Check sheet for the modelled part. Datum: model origin and axes. Units: mm. Face numbers are marked on the shaded views. A direction names the side the tool comes from. Round coordinates to 2 decimals unless told otherwise and drop trailing zeros. Write each loop counter-clockwise with the first axis right and the second up, starting at its lowest first coordinate (ties: lowest second). Pieces come first, ordered by that corner, then holes. Notation, with made-up numbers: (84.25, 59) - (123.25, 59) arc R10 cw to (123.25, 65) - close; hole circle Ø4 at (72.25, -37.5). An arc over 180 degrees is marked (long way). Use one line per item in the form item = value. Start each with the question number.
1) Set-up check for the marked faces 4, 5, 6 and 7: record each of +Z, -Z, +X, -X, +Y, -Y from which the full face is reachable in a straight line by a thin tool's end or side.
2) Draft check along Z on the marked faces 1, 2 and 3. Enter one of: +Z half, -Z half, draft (parallel to the pull), parting line (faces both ways), or undercut.
3) Scan lines: probe 1 along Y at (x, z) = (9, -7.5); probe 2 along Z at (x, y) = (8.25, -28.5); probe 3 along Y at (x, z) = (9.5, -18). Record each from-to range of solid material in increasing order.
4) Gauge pin test, flat ends, axial feed: P1, Ø4.5, axis at x = 10.5, y = -19.5, coming from the +Z side; P2, Ø1.6, axis at y = -25, z = -37.5, coming from the +X side; P3, Ø5, axis at x = 11.5, z = -32, coming from the +Y side; P4, Ø2, axis at x = 5, y = -27, coming from the -Z side. Record the tip position at first contact, or that the pin passes through.
5) Section check C-C (y = 6.5). Record the boundary of the cut face in (x, z).
6) Section check A-A (y = -25). Count the separate pieces of the cut face and the enclosed holes in it, then the cut area to 3 significant figures.
7) Section check B-B (z = -7.5). Record the boundary of the cut face in (x, y), then the cut area to 3 significant figures.
from build123d import *

# Parameters (mm, degrees)
SKETCH_3_W               = 45
SKETCH_3_H               = 5
EXTRUDE_2_DEPTH          = 15
SKETCH_4_W               = 15
SKETCH_4_H               = 5
EXTRUDE_3_DEPTH          = 10
SKETCH_6_R               = 1.25
CUT_EXTRUDE_3_DEPTH      = 50
FILLET_3_R               = 3
SKETCH_7_W               = 15
SKETCH_7_H               = 5
EXTRUDE_4_DEPTH          = 40
FILLET_4_R               = 10
FILLET_5_R               = 5
FILLET_6_R               = 1
FILLET_7_SIZE            = 10
FILLET_7_SIZE_2          = 2.5
SKETCH_8_R               = 1
CUT_EXTRUDE_4_DEPTH      = 40
MIRROR_2_COPY_1_SKETCH_R = 1
MIRROR_2_COPY_1_DEPTH    = 40
MIRROR_2_COPY_2_SKETCH_R = 1
MIRROR_2_COPY_2_DEPTH    = 40
MIRROR_2_COPY_3_SKETCH_R = 1
MIRROR_2_COPY_3_DEPTH    = 40


with BuildPart() as part:
    # 草图3 → 凸台-拉伸2 (new body)
    with BuildSketch(Plane(origin=(0, 0, 0), x_dir=(0, 0, -1), z_dir=(1, 0, 0))):
        with Locations((22.5, 2.5)):
            Rectangle(SKETCH_3_W, SKETCH_3_H)
    extrude(amount=EXTRUDE_2_DEPTH)

    # 草图4 → 凸台-拉伸3 (add)
    with BuildSketch(Plane(origin=(0, 5, 0), x_dir=(1, 0, 0), z_dir=(0, 1, 0))):
        with Locations((7.5, 42.5)):
            Rectangle(SKETCH_4_W, SKETCH_4_H)
        with Locations((7.5, 2.5)):
            Rectangle(SKETCH_4_W, SKETCH_4_H)
    extrude(amount=EXTRUDE_3_DEPTH)

    # 草图6 → 切除-拉伸3 (cut)
    with BuildSketch(Plane.XY):
        with Locations((3.5, 10)):
            Circle(SKETCH_6_R)
        with Locations((11.5, 10)):
            Circle(SKETCH_6_R)
    extrude(amount=-CUT_EXTRUDE_3_DEPTH, mode=Mode.SUBTRACT)

    # 圆角3
    fillet_3_edges = [part.edges().sort_by_distance(p)[0] for p in [
        (0, 15, -42.5),
        (15, 15, -42.5),
        (0, 15, -2.5),
        (15, 15, -2.5),
    ]]
    fillet(fillet_3_edges, radius=FILLET_3_R)

    # 草图7 → 凸台-拉伸4 (add)
    with BuildSketch(Plane(origin=(0, 0, 0), x_dir=(-1, 0, 0), z_dir=(0, -1, 0))):
        with Locations((-7.5, 27.5)):
            Rectangle(SKETCH_7_W, SKETCH_7_H)
        with Locations((-7.5, 17.5)):
            Rectangle(SKETCH_7_W, SKETCH_7_H)
        with Locations((-7.5, 37.5)):
            Rectangle(SKETCH_7_W, SKETCH_7_H)
        with Locations((-7.5, 7.5)):
            Rectangle(SKETCH_7_W, SKETCH_7_H)
    extrude(amount=EXTRUDE_4_DEPTH)

    # 圆角4
    # the kernel refuses this fillet: 10 mm, written as the material it adds along each edge
    with BuildSketch(Plane(origin=(0, 0, -5), x_dir=(0, 0, 1), z_dir=(1, 0, 0)), Plane(origin=(15, 0, -40), x_dir=(0, 0, -1), z_dir=(-1, 0, 0))) as fillet_4_piece_1:
        with BuildLine():
            CenterArc((10, 8.660254038), FILLET_4_R, 180, 60)
            Line((0, 8.660254038), (-0.2, 8.660254038))
            Line((-0.2, 8.660254038), (-0.2, 0))
            Line((-0.2, 0), (0, -0.2))
            ThreePointArc((0, -0.2), (2.5, -0.2), (4.9, -0.173205081))
            Line((4.9, -0.173205081), (5, 0))
        make_face()
    extrude(amount=15)

    # 圆角5
    fillet_5_edges = [part.edges().sort_by_distance(p)[0] for p in [
        (7.5, 0, -45),
        (7.5, 0, 0),
    ]]
    fillet(fillet_5_edges, radius=FILLET_5_R)

    # 圆角6
    fillet_6_edges = [part.edges().sort_by_distance(p)[0] for p in [
        (7.5, -40, -15),
        (7.5, -40, -20),
        (7.5, -40, -35),
        (7.5, -40, -40),
        (7.5, -40, -5),
        (7.5, -40, -10),
        (7.5, -40, -25),
        (7.5, -40, -30),
    ]]
    fillet(fillet_6_edges, radius=FILLET_6_R)

    # 圆角7
    # an asymmetric fillet: 10, 2.5 mm, written as the material it adds along each edge
    with BuildSketch(Plane(origin=(15, 0, -10), x_dir=(0, -1, 0), z_dir=(-1, 0, 0)), Plane(origin=(15, 0, -20), x_dir=(0, -1, 0), z_dir=(-1, 0, 0)), Plane(origin=(15, 0, -30), x_dir=(0, -1, 0), z_dir=(-1, 0, 0)), Plane(origin=(0, 0, -35), x_dir=(0, -1, 0), z_dir=(1, 0, 0))) as fillet_7_piece_1:
        with BuildLine():
            Bezier((FILLET_7_SIZE, 0), (0, 0), (0, -FILLET_7_SIZE_2), weights=[1, 0.707106781, 1])
            Line((0, -FILLET_7_SIZE_2), (0, 0))
            Line((0, 0), (FILLET_7_SIZE, 0))
        make_face()
    extrude(amount=15)
    with BuildSketch(Plane(origin=(0, 0, -15), x_dir=(0, 0, 1), z_dir=(1, 0, 0)), Plane(origin=(0, 0, -25), x_dir=(0, 0, 1), z_dir=(1, 0, 0))) as fillet_7_piece_2:
        with BuildLine():
            Bezier((FILLET_7_SIZE_2, 0), (0, 0), (0, FILLET_7_SIZE), weights=[1, 0.707106781, 1])
            Line((0, FILLET_7_SIZE), (0, 0))
            Line((0, 0), (FILLET_7_SIZE_2, 0))
        make_face()
    extrude(amount=15)

    # 草图8 → 切除-拉伸4 (cut)
    with BuildSketch(Plane.ZY):
        with Locations((-27.5, -15)):
            Circle(SKETCH_8_R)
        with Locations((-27.5, -20)):
            Circle(SKETCH_8_R)
        with Locations((-27.5, -25)):
            Circle(SKETCH_8_R)
        with Locations((-27.5, -30)):
            Circle(SKETCH_8_R)
        with Locations((-27.5, -35)):
            Circle(SKETCH_8_R)
    cut_extrude_4 = extrude(amount=-CUT_EXTRUDE_4_DEPTH, mode=Mode.SUBTRACT)

    # 镜向1: 切除-拉伸4 across plane
    add(cut_extrude_4.mirror(Plane(origin=(0, 0, -32.5), x_dir=(1, 0, 0), z_dir=(0, 0, -1))), mode=Mode.SUBTRACT)

    # 镜向1 at the second plane: 切除-拉伸4 across plane
    add(cut_extrude_4.mirror(Plane(origin=(0, 0, -22.5), x_dir=(1, 0, 0), z_dir=(0, 0, -1))), mode=Mode.SUBTRACT)

    # 镜向2 copy 1 sketch → 镜向2 copy 1 (cut)
    with BuildSketch(Plane(origin=(0, 0, 20), x_dir=(0, 0, 1), z_dir=(-1, 0, 0))):
        with Locations((-27.5, -15)):
            Circle(MIRROR_2_COPY_1_SKETCH_R)
        with Locations((-27.5, -20)):
            Circle(MIRROR_2_COPY_1_SKETCH_R)
        with Locations((-27.5, -25)):
            Circle(MIRROR_2_COPY_1_SKETCH_R)
        with Locations((-27.5, -30)):
            Circle(MIRROR_2_COPY_1_SKETCH_R)
        with Locations((-27.5, -35)):
            Circle(MIRROR_2_COPY_1_SKETCH_R)
    extrude(amount=-MIRROR_2_COPY_1_DEPTH, mode=Mode.SUBTRACT)

    # 镜向2 copy 2 sketch → 镜向2 copy 2 (cut)
    with BuildSketch(Plane.ZY):
        with Locations((-27.5, -15)):
            Circle(MIRROR_2_COPY_2_SKETCH_R)
        with Locations((-27.5, -20)):
            Circle(MIRROR_2_COPY_2_SKETCH_R)
        with Locations((-27.5, -25)):
            Circle(MIRROR_2_COPY_2_SKETCH_R)
        with Locations((-27.5, -30)):
            Circle(MIRROR_2_COPY_2_SKETCH_R)
        with Locations((-27.5, -35)):
            Circle(MIRROR_2_COPY_2_SKETCH_R)
    extrude(amount=-MIRROR_2_COPY_2_DEPTH, mode=Mode.SUBTRACT)

    # 镜向2 copy 3 sketch → 镜向2 copy 3 (cut)
    with BuildSketch(Plane(origin=(0, 0, -45), x_dir=(0, 0, -1), z_dir=(-1, 0, 0))):
        with Locations((-27.5, 15)):
            Circle(MIRROR_2_COPY_3_SKETCH_R)
        with Locations((-27.5, 20)):
            Circle(MIRROR_2_COPY_3_SKETCH_R)
        with Locations((-27.5, 25)):
            Circle(MIRROR_2_COPY_3_SKETCH_R)
        with Locations((-27.5, 30)):
            Circle(MIRROR_2_COPY_3_SKETCH_R)
        with Locations((-27.5, 35)):
            Circle(MIRROR_2_COPY_3_SKETCH_R)
    extrude(amount=-MIRROR_2_COPY_3_DEPTH, mode=Mode.SUBTRACT)


solid = part.part
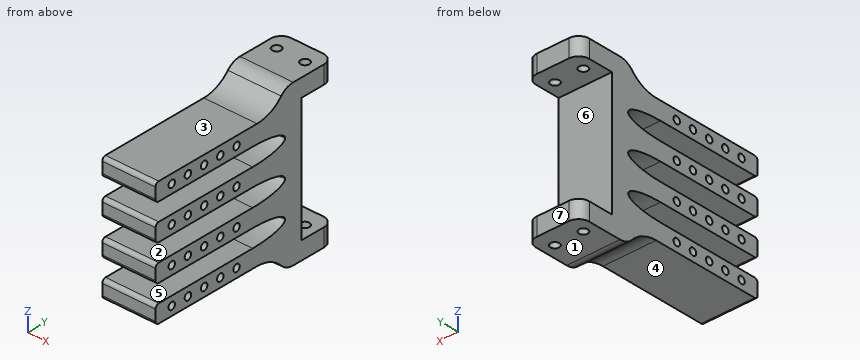
Results are:
q1.face_4 = -Z, +X, -X, -Y
q1.face_5 = +X, -X, -Y
q1.face_6 = +X, -X, +Y
q1.face_7 = +Z, -Z, +X, -X, +Y
q2.face_1 = -Z half
q2.face_2 = undercut
q2.face_3 = +Z half
q3.probe_1 = -40 to -36, -34 to -31, -29 to -26, -24 to -21, -19 to -16, -14 to 5
q3.probe_2 = -40 to -35, -30 to -25, -20 to -15, -10 to -5
q3.probe_3 = -40 to -35.87, -34.13 to -30.87, -29.13 to -25.87, -24.13 to -20.87, -19.13 to -15.87, -14.13 to 5
q4.P1 = -5
q4.P2 = through
q4.P3 = 5
q4.P4 = -40
q5.outline = (0, -45) - (15, -45) - (15, -40) - (0, -40) - close; (0, -5) - (15, -5) - (15, 0) - (0, 0) - close
q6.separate_pieces = 8
q6.enclosed_holes = 0
q6.area = 180 mm²
q7.outline = (0, -40) - (15, -40) - (15, -36) - (0, -36) - close; (0, -34) - (15, -34) - (15, -31) - (0, -31) - close; (0, -29) - (15, -29) - (15, -26) - (0, -26) - close; (0, -24) - (15, -24) - (15, -21) - (0, -21) - close; (0, -19) - (15, -19) - (15, -16) - (0, -16) - close; (0, -14) - (15, -14) - (15, 5) - (0, 5) - close
q7.area = 525 mm²
